Source: three-view drawing plus pictorial views. Frame: mm from the lowest corner of the part. A direction names the side the tool comes from. Coordinates: 2 decimals unless noted, no trailing zeros. Order: outer loops, then holes, each group sorted by start corner. A loop starts at its lowest first (then second) coordinate and runs counter-clockwise, first axis right, second up. Notation, with made-up numbers: (20, 25) -> (45, 25) arc R21 ccw to (45, 31) -> close; hole circle Ø5 at (24, -9). An arc over 180 degrees is marked (long way). Use one line per item in the form item = value. Start each with the question number.
1) Section query C-C on y = 6. Output: boundary loops of the cut face in (x, z), then the cut area to 3 significant figures.
2) Access query for the marked faces 1, 2 and 3. Directions: +Z, -Z, +X, -X, +Y, -Y. A direction counts if a zero-diameter tool reaches every point of the face in a straight line with its end or side. Return the directions, or none.
3) Section query D-D on x = 33. Output: boundary loops of the cut face in (y, z), then the cut area to 3 significant figures.
4) Draft query along X for the marked faces 4, 5, 6 and 7. Return one class per face: pulls with the +X half, pulls with the -X half, needs draft (parallel to the pull), parting line crosses it, or undercut.
5) Pin query (flat end, axial travel): pin 1 (1 mm diameter, centred on x = 14.5, y = 28.5, fed in from -Z); pin 2 (2 mm diameter, centred on x = 18, z = 1.5, fed in from +Y). Return the tip coordinate at first contact, or that it passes through.
6) Section query A-A on y = 33.5. Output: boundary loops of the cut face in (x, z).
7) Section query B-B on z = 3.55. Output: boundary loops of the cut face in (x, y).
8) Ray query, line 1 along X through (y, z) = (27, 4.3); line 2 along X through (y, z) = (6, 1.3); line 3 along Y through (x, z) = (20, 1.2). Return the intervals inside material, ascending.
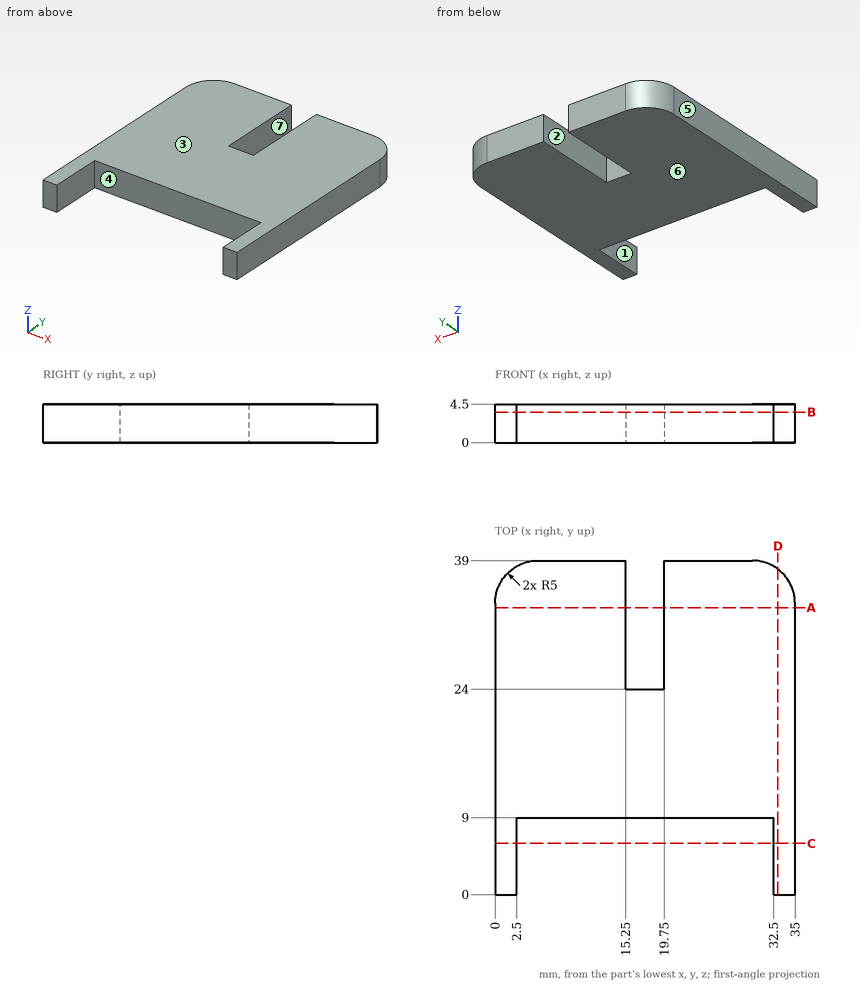
Answers below:
q1.outline = (0, 0) -> (2.5, 0) -> (2.5, 4.5) -> (0, 4.5) -> close; (32.5, 0) -> (35, 0) -> (35, 4.5) -> (32.5, 4.5) -> close
q1.area = 22.5 mm^2
q2.face_1 = +Z, -Z, -Y
q2.face_2 = +Z, -Z, +Y
q2.face_3 = +Z, +X, -X, +Y, -Y
q3.outline = (0, 0) -> (38, 0) -> (38, 4.5) -> (0, 4.5) -> close
q3.area = 171 mm^2
q4.face_4 = undercut
q4.face_5 = pulls with the -X half
q4.face_6 = needs draft
q4.face_7 = undercut
q5.pin_1 = 0
q5.pin_2 = 24
q6.outline = (0, 0) -> (15.25, 0) -> (15.25, 4.5) -> (0, 4.5) -> close; (19.75, 0) -> (35, 0) -> (35, 4.5) -> (19.75, 4.5) -> close
q7.outline = (0, 0) -> (2.5, 0) -> (2.5, 9) -> (32.5, 9) -> (32.5, 0) -> (35, 0) -> (35, 34) arc R5 ccw to (30, 39) -> (19.75, 39) -> (19.75, 24) -> (15.25, 24) -> (15.25, 39) -> (5, 39) arc R5 ccw to (0, 34) -> close
q8.line_1 = 0 to 15.25, 19.75 to 35
q8.line_2 = 0 to 2.5, 32.5 to 35
q8.line_3 = 9 to 39
